```python
from build123d import *

# Parameters (mm, degrees)
F3_R = 3


with BuildPart() as f2:
    # F2: sweep along a path in F1
    with BuildLine(Plane.YZ) as f2_path:
        Line((0, 0), (0, 30))
        Line((0, 30), (-38.5672565812, 75.9626665871))
        Line((-38.5672565812, 75.9626665871), (-68.1114891716, 81.1721119171))
    # F0 (on Top) → F2 (sweep)
    with BuildSketch(Plane.XY):
        with BuildLine():
            Line((-10, 15), (-20, 15))
            Line((-20, 15), (-20, -15))
            Line((-20, -15), (20, -15))
            Line((20, -15), (20, 15))
            Line((20, 15), (10, 15))
            add(Edge.make_bspline(
                [(10, 15), (12.8331761755, 9.8207678803), (17.947046752, 0.4722766093), (10.6957463234, -10.4813852615), (3.5543120142, -10.4875882246), (0, -10.4906754568)],
                knots=[0, 0, 0, 0, 0.3842269917, 0.6935280356, 1, 1, 1, 1], degree=3))
            add(Edge.make_bspline(
                [(-10, 15), (-12.8331761755, 9.8207678803), (-17.947046752, 0.4722766093), (-10.6957463234, -10.4813852615), (-3.5543120142, -10.4875882246), (0, -10.4906754568)],
                knots=[0, 0, 0, 0, 0.3842269917, 0.6935280356, 1, 1, 1, 1], degree=3))
        make_face()
    sweep(path=f2_path.line, transition=Transition.RIGHT)

    # F3
    f3_edges = [f2.edges().sort_by_distance(p)[0] for p in [
        (-20, 15, 17.729777),
        (-20, -7.792962, 62.623147),
        (-20, -48.046345, 92.865485),
        (-20, -68.111489, 81.172112),
        (-20, -58.632401, 64.269294),
        (-20, -30.774295, 43.339519),
        (-20, -15, 12.270223),
        (-20, 0, 0),
        (20, -48.046345, 92.865485),
        (20, -7.792962, 62.623147),
        (20, 15, 17.729777),
        (20, 0, 0),
        (20, -15, 12.270223),
        (20, -30.774295, 43.339519),
        (20, -58.632401, 64.269294),
        (20, -68.111489, 81.172112),
    ]]
    fillet(f3_edges, radius=F3_R)


solid = f2.part
```
Work out the finished part from the listing and answer in its coordinate system (mm). A direction names the side the tool comes from. Give positions to 0.01 mm unless a question says otherwise; leave off trailing zeros. One line per item, written item: value. Start each with the question number.
1. Which of the six approach directions +Z, -Z, +X, -X, +Y, -Y give full straight-line access (tool end or side, diameter ignored) to faces 1 (the face through (19.1, -14.14, 13)), 2 (the face through (0, -15, 12)), 3 (the face through (-19.14, -14.1, 13))?
2. Each of these flat-tipped pins is pushed along its axis until it touches: P1, Ø6, axis at x = -6.5, z = 49, coming from the -Y side; P2, Ø1.5, axis at x = 12, z = 78, coming from the +Y side; P3, Ø8, axis at x = -14.5, y = -51, coming from the -Z side. Where does it stop, or does it pass through?
3. Find the intervals of material crossed by probe 1 along X at (y, z) = (5.5, 35.5); probe 2 along X at (y, z) = (-28, 78); probe 3 along Y at (x, z) = (-11.5, 11.5), in increasing order.
Reported:
1. face 1: -Z, +X, -Y
1. face 2: -Z, +X, -X, -Y
1. face 3: -Z, -X, -Y
2. P1: stops at y = -38.04
2. P2: stops at y = -20.07
2. P3: stops at z = 62.22
3. probe 1: x = -20 to -13.67, 13.67 to 20
3. probe 2: x = -20 to -12.93, 12.93 to 20
3. probe 3: y = -15 to -7.75, 12.23 to 15
